Verification items for the finished model (mm, model axes). A direction names the side the tool comes from. Give positions to 0.01 mm unless a question says otherwise; leave off trailing zeros. Loops run counter-clockwise (first coordinate to the right, second up) from the corner with the lowest first, then second, coordinate; pieces in that order, holes last. Notation, with made-up numbers: M -16,-11 L 43,-11 A31 ccw 43,27 Z; hole C -24.75,36.25 d10. An arc over 180 degrees is marked long. Use a Markdown table: item, result.
from build123d import *

# Parameters (mm, degrees)
SKETCH1_W           = 40
SKETCH1_H           = 40
BOSS_EXTRUDE1_DEPTH = 3
SKETCH2_R           = 1.65
CUT_EXTRUDE1_DEPTH  = 3
SKETCH3_W           = 40
SKETCH3_H           = 3
BOSS_EXTRUDE2_DEPTH = 3
SKETCH4_W           = 40
SKETCH4_H           = 50.5
BOSS_EXTRUDE3_DEPTH = 3


with BuildPart() as part:
    # Sketch1 → Boss-Extrude1 (new body)
    with BuildSketch(Plane.XY):
        with Locations((20, 20)):
            Rectangle(SKETCH1_W, SKETCH1_H)
    extrude(amount=BOSS_EXTRUDE1_DEPTH)

    # Sketch2 → Cut-Extrude1 (cut)
    with BuildSketch(Plane.XY.offset(3)):
        with Locations((3.5, 36.5)):
            Circle(SKETCH2_R)
        with Locations(Location((36.5, 36.5, 0), (0, 0, 180))):
            Circle(SKETCH2_R)
        with Locations((36.5, 3.5)):
            Circle(SKETCH2_R)
        with Locations(Location((3.5, 3.5, 0), (0, 0, 180))):
            Circle(SKETCH2_R)
    extrude(amount=-CUT_EXTRUDE1_DEPTH, mode=Mode.SUBTRACT)

    # Sketch3 → Boss-Extrude2 (add)
    with BuildSketch(Plane.XY.offset(3)):
        with Locations((20, -1.5)):
            Rectangle(SKETCH3_W, SKETCH3_H)
    extrude(amount=-BOSS_EXTRUDE2_DEPTH)

    # Sketch4 → Boss-Extrude3 (add)
    with BuildSketch(Plane.XZ.offset(3)):
        with Locations((20, 28.25)):
            Rectangle(SKETCH4_W, SKETCH4_H)
        with BuildLine():
            Line((7.28, 50.5), (10.2, 50.5))
            Line((10.2, 50.5), (10.2, 47.3))
            ThreePointArc((10.2, 47.3), (11.6, 45.9), (10.2, 44.5))
            Line((10.2, 44.5), (7.28, 44.5))
            Line((7.28, 44.5), (7.28, 50.5))
        make_face(mode=Mode.SUBTRACT)
        with BuildLine():
            Line((32.72, 50.5), (32.72, 44.5))
            Line((32.72, 44.5), (29.8, 44.5))
            ThreePointArc((29.8, 44.5), (28.4, 45.9), (29.8, 47.3))
            Line((29.8, 47.3), (29.8, 50.5))
            Line((29.8, 50.5), (32.72, 50.5))
        make_face(mode=Mode.SUBTRACT)
        with BuildLine():
            Line((32.72, 6), (29.8, 6))
            Line((29.8, 6), (29.8, 9.2))
            ThreePointArc((29.8, 9.2), (28.4, 10.6), (29.8, 12))
            Line((29.8, 12), (32.72, 12))
            Line((32.72, 12), (32.72, 6))
        make_face(mode=Mode.SUBTRACT)
        with BuildLine():
            Line((7.28, 6), (7.28, 12))
            Line((7.28, 12), (10.2, 12))
            ThreePointArc((10.2, 12), (11.6, 10.6), (10.2, 9.2))
            Line((10.2, 9.2), (10.2, 6))
            Line((10.2, 6), (7.28, 6))
        make_face(mode=Mode.SUBTRACT)
    extrude(amount=-BOSS_EXTRUDE3_DEPTH)


solid = part.part
(1) Draft check along Z on faces 3 (the flat face through (20, 20, 3)), 4 (the cylindrical face through (4.39, 37.89, 1.52)), 5 (the flat face through (9, -2, 12)). Enter one of: +Z half, -Z half, draft (parallel to the pull), parting line (faces both ways), or undercut.
Results below:
| item | result |
|---|---|
| face 3 | +Z half |
| face 4 | draft |
| face 5 | undercut |
(2) Gauge pin test, flat end, axial feed: P1, Ø6, axis at x = 29.5, y = 23.5, coming from the +Z side. Record the tip position at first contact, or that the pin passes through.
Results below:
| item | result |
|---|---|
| P1 | z = 3 |
(3) Cross-section at D-D on y = 9. Record the cut outline in (x, z).
Results below:
| item | result |
|---|---|
| outline | M 0,0 L 40,0 L 40,3 L 0,3 Z |
(4) Cross-section at B-B on z = 45.9. Record the cut outline in (x, y), then the cut area to 3 significant figures.
Results below:
| item | result |
|---|---|
| outline | M 0,-3 L 7.28,-3 L 7.28,0 L 0,0 Z; M 11.6,-3 L 28.4,-3 L 28.4,0 L 11.6,0 Z; M 32.72,-3 L 40,-3 L 40,0 L 32.72,0 Z |
| area | 94.1 mm^2 |
(5) Cross-section at A-A on x = 36.5. Record the cut outline in (y, z), then the cut area to 3 significant figures.
Results below:
| item | result |
|---|---|
| outline | M -3,0 L 1.85,0 L 1.85,3 L 0,3 L 0,53.5 L -3,53.5 Z; M 5.15,0 L 34.85,0 L 34.85,3 L 5.15,3 Z; M 38.15,0 L 40,0 L 40,3 L 38.15,3 Z |
| area | 261 mm^2 |
(6) Material ranges on line 1 (Y direction, x = 36.5, z = 1.95); line 2 (X direction, y = 36, z = 2); line 3 (Z direction, x = 23.5, y = 19), recorded low to high.
Results below:
| item | result |
|---|---|
| line 1 | -3 to 1.85, 5.15 to 34.85, 38.15 to 40 |
| line 2 | 0 to 1.93, 5.07 to 34.93, 38.07 to 40 |
| line 3 | 0 to 3 |
(7) Cross-section at C-C on x = 6. Record the cut outline in (y, z), then the cut area to 4 significant figures.
Results below:
| item | result |
|---|---|
| outline | M -3,0 L 40,0 L 40,3 L 0,3 L 0,53.5 L -3,53.5 Z |
| area | 280.5 mm^2 |
(8) Set-up check for faces 1 (the cylindrical face through (3.9, 5.1, 1.5)), 2 (the cylindrical face through (28.4, -1.5, 10.6)): record each of +Z, -Z, +X, -X, +Y, -Y from which the full face is reachable in a straight line by a thin tool's end or side.
Results below:
| item | result |
|---|---|
| face 1 | +Z, -Z |
| face 2 | +Y, -Y |
